Autodesk Inventor part; units mm, degrees
ref_plane "YZ Plane" through (0, 0, 0) normal (1, 0, 0) x (0, 1, 0)
ref_plane "XZ Plane" through (0, 0, 0) normal (0, 1, 0) x (-1, 0, 0)
ref_plane "XY Plane" through (0, 0, 0) normal (0, 0, 1) x (1, 0, 0)
sketch "Sketch1" plane through (0, 0, 0) normal (0, 0, 1) x (1, 0, 0)
  line L0 (90.332, 117.5659) -> (90.332, 153.0357)
  line L1 (88.4722, 157.5258) -> (66.7919, 179.2061)
  line L2 (62.3018, 181.0659) -> (-138.268, 181.0659)
  circle A0 centre (60.8045, 142.9659) radius 14.2875
  arc A1 (66.7919, 179.2061) -> (62.3018, 181.0659) centre (62.3018, 174.7159) ccw
  arc A2 (90.332, 153.0357) -> (88.4722, 157.5258) centre (83.982, 153.0357) ccw
  arc A3 (83.982, 111.2159) -> (90.332, 117.5659) centre (83.982, 117.5659) ccw
  line L3 (-138.268, 111.2159) -> (83.982, 111.2159)
  arc A4 (-138.268, 181.0659) -> (-138.268, 111.2159) centre (-138.268, 146.1409) ccw
  circle A5 centre (-138.268, 146.1409) radius 3.175
  dimension "d61" = 69.85
  dimension "d68" = 222.25
  dimension "d69" = 200.5697
  dimension "d71" = 28.575
  dimension "d72" = 6.35
extrude "Extrusion10" add sketch "Sketch1" along normal blind 12.7
sketch "Sketch8" plane through (0, 0, 12.7) normal (0, 0, 1) x (1, 0, 0)
  circle A0 centre (60.8045, 142.9659) radius 14.2875
  circle A1 centre (-138.268, 146.1409) radius 3.175
  line L0 (62.3018, 181.0659) -> (-138.268, 181.0659)
  arc A2 (-138.268, 181.0659) -> (-138.268, 111.2159) centre (-138.268, 146.1409) ccw
  line L1 (-138.268, 111.2159) -> (83.982, 111.2159)
  arc A3 (83.982, 111.2159) -> (90.332, 117.5659) centre (83.982, 117.5659) ccw
  line L2 (90.332, 117.5659) -> (90.332, 153.0357)
  arc A4 (90.332, 153.0357) -> (88.4722, 157.5258) centre (83.982, 153.0357) ccw
  line L3 (88.4722, 157.5258) -> (66.7919, 179.2061)
  arc A5 (66.7919, 179.2061) -> (62.3018, 181.0659) centre (62.3018, 174.7159) ccw
  circle A6 centre (60.8045, 142.9659) radius 50.8 construction
  line L4 (60.8045, 142.9659) -> (-28.0955, 142.9659) construction
  circle A7 centre (-28.0955, 142.9659) radius 14.2875
  point P0 (0, 0)
  dimension "d75" = 101.6
  dimension "d76" = 88.9
  dimension "d77" = 28.575
extrude "Extrusion11" cut sketch "Sketch8" against normal through all contours A7
sketch "Sketch9" plane through (0, 0, 12.7) normal (0, 0, 1) x (1, 0, 0)
  circle A0 centre (-28.0955, 142.9659) radius 14.2875
  circle A1 centre (60.8045, 142.9659) radius 14.2875
  circle A2 centre (-138.268, 146.1409) radius 3.175
  line L0 (62.3018, 181.0659) -> (-138.268, 181.0659)
  arc A3 (-138.268, 181.0659) -> (-138.268, 111.2159) centre (-138.268, 146.1409) ccw
  line L1 (-138.268, 111.2159) -> (83.982, 111.2159)
  arc A4 (83.982, 111.2159) -> (90.332, 117.5659) centre (83.982, 117.5659) ccw
  line L2 (90.332, 117.5659) -> (90.332, 153.0357)
  arc A5 (90.332, 153.0357) -> (88.4722, 157.5258) centre (83.982, 153.0357) ccw
  line L3 (88.4722, 157.5258) -> (66.7919, 179.2061)
  arc A6 (66.7919, 179.2061) -> (62.3018, 181.0659) centre (62.3018, 174.7159) ccw
  line L4 (60.8045, 142.9659) -> (111.6045, 142.9659)
  line L5 (-173.193, 146.1409) -> (-173.193, 114.3909)
  line L6 (60.8045, 142.9659) -> (-173.193, 142.9659)
  point P0 (0, 0)
  dimension "d80" = 50.8
  dimension "d81" = 284.7975
sketch "Sketch10" plane through (0, 0, 12.7) normal (0, 0, 1) x (1, 0, 0)
  circle A0 centre (-28.0955, 142.9659) radius 14.2875
  circle A1 centre (60.8045, 142.9659) radius 14.2875
  circle A2 centre (-138.268, 146.1409) radius 3.175
  line L0 (62.3018, 181.0659) -> (-138.268, 181.0659)
  arc A3 (-138.268, 181.0659) -> (-138.268, 111.2159) centre (-138.268, 146.1409) ccw
  line L1 (-138.268, 111.2159) -> (83.982, 111.2159)
  arc A4 (83.982, 111.2159) -> (90.332, 117.5659) centre (83.982, 117.5659) ccw
  line L2 (90.332, 117.5659) -> (90.332, 153.0357)
  arc A5 (90.332, 153.0357) -> (88.4722, 157.5258) centre (83.982, 153.0357) ccw
  line L3 (88.4722, 157.5258) -> (66.7919, 179.2061)
  arc A6 (66.7919, 179.2061) -> (62.3018, 181.0659) centre (62.3018, 174.7159) ccw
  line L4 (-138.268, 146.1409) -> (-87.468, 146.1409) construction
  circle A7 centre (-87.468, 146.1409) radius 3.175
  point P0 (0, 0)
  dimension "d82" = 50.8
  dimension "d83" = 6.35
extrude "Extrusion12" cut sketch "Sketch10" against normal through all contours A7
properties part number "Top IntakeBar"
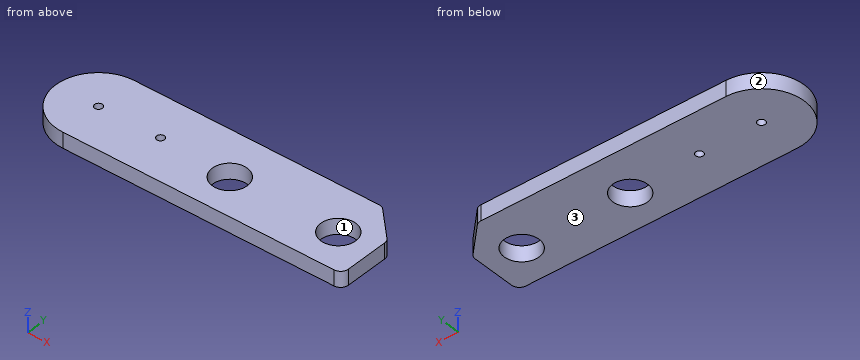
Geometry: final body of the model. Coordinates: model frame, mm. Face numbers are marked on the shaded views. Coordinates: 2 decimals unless noted, no trailing zeros. Write each loop counter-clockwise with the first axis right and the second up, starting at its lowest first coordinate (ties: lowest second). Pieces come first, ordered by that corner, then holes. Notation, with made-up numbers: M 33.25,22.25 L 88.25,22.25 A31 cw 88.25,50.25 Z; hole C 43,60 d2. An arc over 180 degrees is marked long. Answer as CSV lines item,"result". Start each with the question number.
Q1. Cut plane D-D on x = -87.5. Return the cut outline in (y, z).
Q2. Mould query, pull axis X, two halves, no side actions, for the marked faces 1, 2 and 3. Classes: released by +X, released by -X, zero draft, split by the parting line, or undercut.
Q3. Cut plane B-B on y = 136. Return the cut outline in (x, z).
Q4. Line query: line 1 (Y direction, x = -87.5, z = 11.5); line 2 (X direction, y = 144.5, z = 11); line 3 (X direction, y = 133.5, z = 9.5). Output: solid intervals per line, ascending. Write a range as from..to.
Q5. Cut plane C-C on z = 4. Count the separate pieces of the cut face and the enclosed holes in it, then the cut area to 3 significant figures.
Q6. Pin query (flat end, axial travel): P1, Ø6, axis at y = 164.5, z = 8.5, coming from the -X side; P2, Ø2, axis at y = 167.5, z = 9, coming from the -X side; P3, Ø23, axis at x = 60.8, y = 142.97, coming from the +Z side; P4, Ø2, axis at y = 123.5, z = 8, coming from the -X side. Return the tip coordinate at first contact, or that it passes through.
Q7. Cut plane A-A on x = 59.5. Return the cut outline in (y, z), then the cut area to 3 significant figures.
Findings below:
1,outline,"M 111.22,0 L 142.97,0 L 142.97,12.7 L 111.22,12.7 Z; M 149.32,0 L 181.07,0 L 181.07,12.7 L 149.32,12.7 Z"
2,face 1,"undercut"
2,face 2,"released by -X"
2,face 3,"zero draft"
3,outline,"M -171.69,0 L -40.57,0 L -40.57,12.7 L -171.69,12.7 Z; M -15.62,0 L 48.33,0 L 48.33,12.7 L -15.62,12.7 Z; M 73.28,0 L 90.33,0 L 90.33,12.7 L 73.28,12.7 Z"
4,line 1,"y = 111.22..142.97, 149.32..181.07"
4,line 2,"x = -173.15..-140.99, -135.55..-90.19, -84.75..-42.3, -13.89..46.6, 75.01..90.33"
4,line 3,"x = -170.83..-38.8, -17.39..50.1, 71.51..90.33"
5,separate pieces,"1"
5,enclosed holes,"4"
5,area,"16,200 mm2"
6,P1,"stops at x = -169.63"
6,P2,"stops at x = -166.65"
6,P3,"passes through"
6,P4,"stops at x = -165.68"
7,outline,"M 111.22,0 L 128.74,0 L 128.74,12.7 L 111.22,12.7 Z; M 157.19,0 L 181.07,0 L 181.07,12.7 L 157.19,12.7 Z"
7,area,"526 mm2"
